```python
from build123d import *

# Parameters (mm, degrees)
SKETCH1_R           = 75
BOSS_EXTRUDE1_DEPTH = 180
SKETCH2_R           = 105
BOSS_EXTRUDE2_DEPTH = 25
SKETCH3_R           = 105
BOSS_EXTRUDE3_DEPTH = 25
FILLET1_R           = 10


with BuildPart() as part:
    # Sketch1 → Boss-Extrude1 (new body)
    with BuildSketch(Plane.XY):
        Circle(SKETCH1_R)
    extrude(amount=BOSS_EXTRUDE1_DEPTH)

    # Sketch2 → Boss-Extrude2 (add)
    with BuildSketch(Plane.XY.offset(180)):
        Circle(SKETCH2_R)
    extrude(amount=BOSS_EXTRUDE2_DEPTH)

    # Sketch3 → Boss-Extrude3 (add)
    with BuildSketch(Plane(origin=(0, 0, 0), x_dir=(-1, 0, 0), z_dir=(0, 0, -1))):
        Circle(SKETCH3_R)
    extrude(amount=BOSS_EXTRUDE3_DEPTH)

    # Fillet1
    fillet1_edges = [part.edges().sort_by_distance(p)[0] for p in [
        (105, 0, -25),
        (-105, 0, 205),
    ]]
    fillet(fillet1_edges, radius=FILLET1_R)


solid = part.part
```
Geometry check sheet. Reference: the model listing, model coordinates, mm. A direction names the side the tool comes from. Coordinates: 2 decimals unless noted, no trailing zeros. Order: outer loops, then holes, each group sorted by start corner. A loop starts at its lowest first (then second) coordinate and runs counter-clockwise, first axis right, second up.
Item 1: Depth check by flat-ended pin: pin 1 (4 mm diameter, centred on x = -64.5, y = -79.5, fed in from +Z); pin 2 (12 mm diameter, centred on y = 36.5, z = 116.5, fed in from +X); pin 3 (5 mm diameter, centred on x = -55, z = 93.5, fed in from +Y). Enter the tip coordinate at first touch or a pass-through.
Item 2: Section check C-C (z = 190.5). Enter the section's corners in (x, y), plus the area to 3 significant figures.
Item 3: Section check A-A (x = 0). Enter the section's corners in (y, z), plus the area to 3 significant figures.
Item 4: Tool access check on faces 1 (the cylindrical face through (100.15, 31.54, 187.4)), 2 (the cylindrical face through (-9.764, 74.362, 88.74)). Record the directions out of +Z, -Z, +X, -X, +Y, -Y that give a thin tool (end or side, any length) a straight path to the whole face; none if there is none.
Item 5: Scan lines: line 1 along Z through (x, y) = (-25, 77); line 2 along X through (y, z) = (-2.5, 149.5); line 3 along Y through (x, z) = (-52.5, 82.5). Record each from-to range of solid material in increasing order.
Item 6: Section check D-D (z = 166). Enter the section's corners in (x, y), plus the area to 3 significant figures.
Check sheet entries:
1. pin 1: stops at z = 203.43
1. pin 2: stops at x = 68.52
1. pin 3: stops at y = 53.56
2. outline: circle Ø210 at (0, 0)
2. area: 34,600 mm2
3. outline: (-105, -15) arc R10 ccw to (-95, -25) - (95, -25) arc R10 ccw to (105, -15) - (105, 0) - (75, 0) - (75, 180) - (105, 180) - (105, 195) arc R10 ccw to (95, 205) - (-95, 205) arc R10 ccw to (-105, 195) - (-105, 180) - (-75, 180) - (-75, 0) - (-105, 0) - close
3. area: 37,400 mm2
4. face 1: +Z, -Z
4. face 2: none
5. line 1: z = -25 to 0, 180 to 205
5. line 2: x = -74.96 to 74.96
5. line 3: y = -53.56 to 53.56
6. outline: circle Ø150 at (0, 0)
6. area: 17,700 mm2
